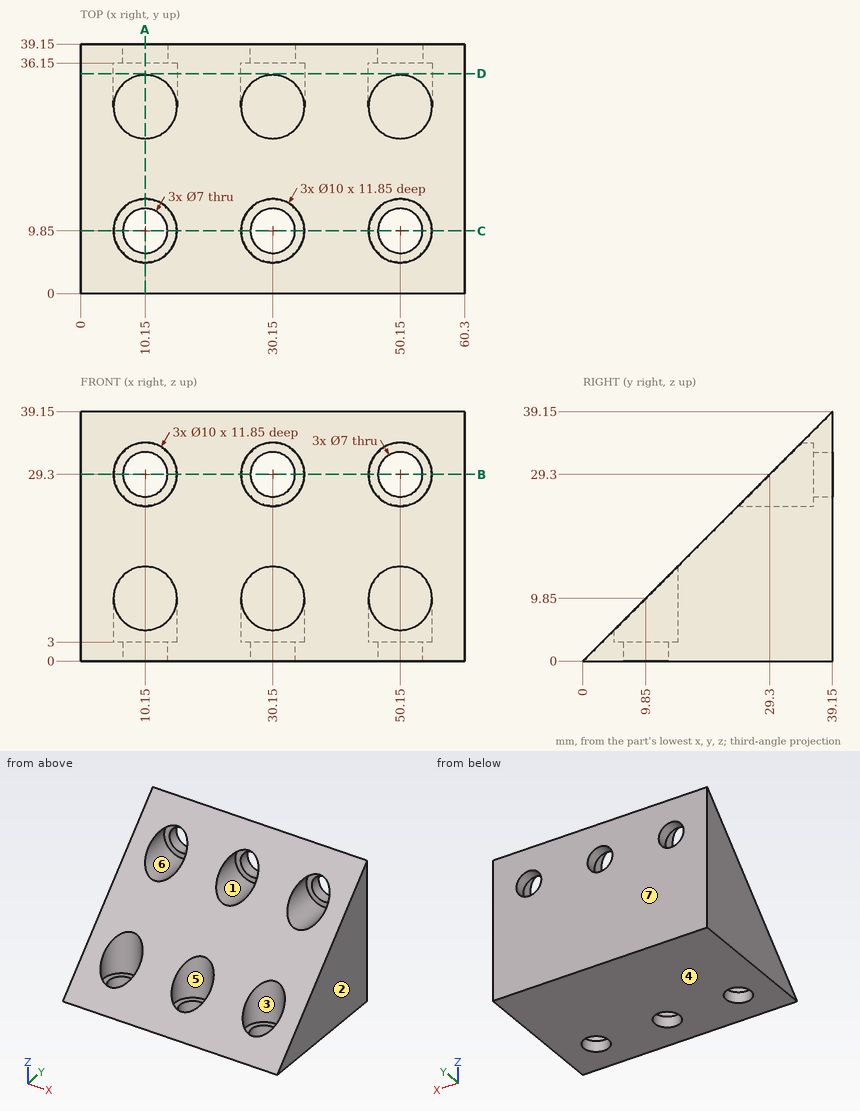
Verification items for this drawing (mm, ordinates from the low corner). A direction names the side the tool comes from. Coordinates: 2 decimals unless noted, no trailing zeros. Order: outer loops, then holes, each group sorted by start corner. A loop starts at its lowest first (then second) coordinate and runs counter-clockwise, first axis right, second up.
Q1. Tool access check on the marked faces 5, 6 and 7. Record the directions out of +Z, -Z, +X, -X, +Y, -Y that give a thin tool (end or side, any length) a straight path to the whole face; none if there is none.
Reply:
face 5: +Z
face 6: -Y
face 7: +Z, -Z, +X, -X, +Y
Q2. Sectioned sample at C-C on y = 9.85. Record the cut outline in (x, z).
Reply:
outline: (0, 0) - (6.65, 0) - (6.65, 3) - (5.15, 3) - (5.15, 9.85) - (0, 9.85) - close; (13.65, 0) - (26.65, 0) - (26.65, 3) - (25.15, 3) - (25.15, 9.85) - (15.15, 9.85) - (15.15, 3) - (13.65, 3) - close; (33.65, 0) - (46.65, 0) - (46.65, 3) - (45.15, 3) - (45.15, 9.85) - (35.15, 9.85) - (35.15, 3) - (33.65, 3) - close; (53.65, 0) - (60.3, 0) - (60.3, 9.85) - (55.15, 9.85) - (55.15, 3) - (53.65, 3) - close
Q3. Depth check by flat-ended pin: pin 1 Ø8 at (x, z) = (50.15, 29.3) entering from +Y; pin 2 Ø8 at (x, z) = (10.15, 29.3) entering from -Y; pin 3 Ø8 at (x, z) = (18, 9) entering from -Y; pin 4 Ø3 at (x, y) = (32.5, 9) entering from +Z. Enter the tip coordinate at first touch or a pass-through.
Reply:
pin 1: stops at y = 39.15
pin 2: stops at y = 36.15
pin 3: stops at y = 5
pin 4: stops at z = 3
Q4. Thickness scan on probe 1 along X at (y, z) = (31, 27.5); probe 2 along X at (y, z) = (13, 5); probe 3 along Y at (x, z) = (26.5, 30). Record the ranges inside material, lowest first.
Reply:
probe 1: x = 0 to 5.49, 14.81 to 25.49, 34.81 to 45.49, 54.81 to 60.3
probe 2: x = 0 to 6.27, 14.03 to 26.27, 34.03 to 46.27, 54.03 to 60.3
probe 3: y = 36.15 to 39.15
Q5. Draft check along X on the marked faces 1, 2, 3 and 4. Enter one of: released by +X, released by -X, zero draft, split by the parting line, or undercut.
Reply:
face 1: undercut
face 2: released by +X
face 3: undercut
face 4: zero draft
Q6. Sectioned sample at B-B on z = 29.3. Record the cut outline in (x, y).
Reply:
outline: (0, 29.3) - (5.15, 29.3) - (5.15, 36.15) - (6.65, 36.15) - (6.65, 39.15) - (0, 39.15) - close; (13.65, 36.15) - (15.15, 36.15) - (15.15, 29.3) - (25.15, 29.3) - (25.15, 36.15) - (26.65, 36.15) - (26.65, 39.15) - (13.65, 39.15) - close; (33.65, 36.15) - (35.15, 36.15) - (35.15, 29.3) - (45.15, 29.3) - (45.15, 36.15) - (46.65, 36.15) - (46.65, 39.15) - (33.65, 39.15) - close; (53.65, 36.15) - (55.15, 36.15) - (55.15, 29.3) - (60.3, 29.3) - (60.3, 39.15) - (53.65, 39.15) - close
Q7. Sectioned sample at A-A on x = 10.15. Record the cut outline in (y, z).
Reply:
outline: (0, 0) - (6.35, 0) - (6.35, 3) - (4.85, 3) - (4.85, 4.85) - close; (13.35, 0) - (39.15, 0) - (39.15, 25.8) - (36.15, 25.8) - (36.15, 24.3) - (24.3, 24.3) - (14.85, 14.85) - (14.85, 3) - (13.35, 3) - close; (34.3, 34.3) - (36.15, 34.3) - (36.15, 32.8) - (39.15, 32.8) - (39.15, 39.15) - close
Q8. Sectioned sample at D-D on y = 34.5. Record the cut outline in (x, z), and give its area (3 significant figures).
Reply:
outline: (0, 0) - (60.3, 0) - (60.3, 34.5) - (0, 34.5) - close; hole circle Ø10 at (10.15, 29.3); hole circle Ø10 at (30.15, 29.3); hole circle Ø10 at (50.15, 29.3)
area: 1,840 mm2
